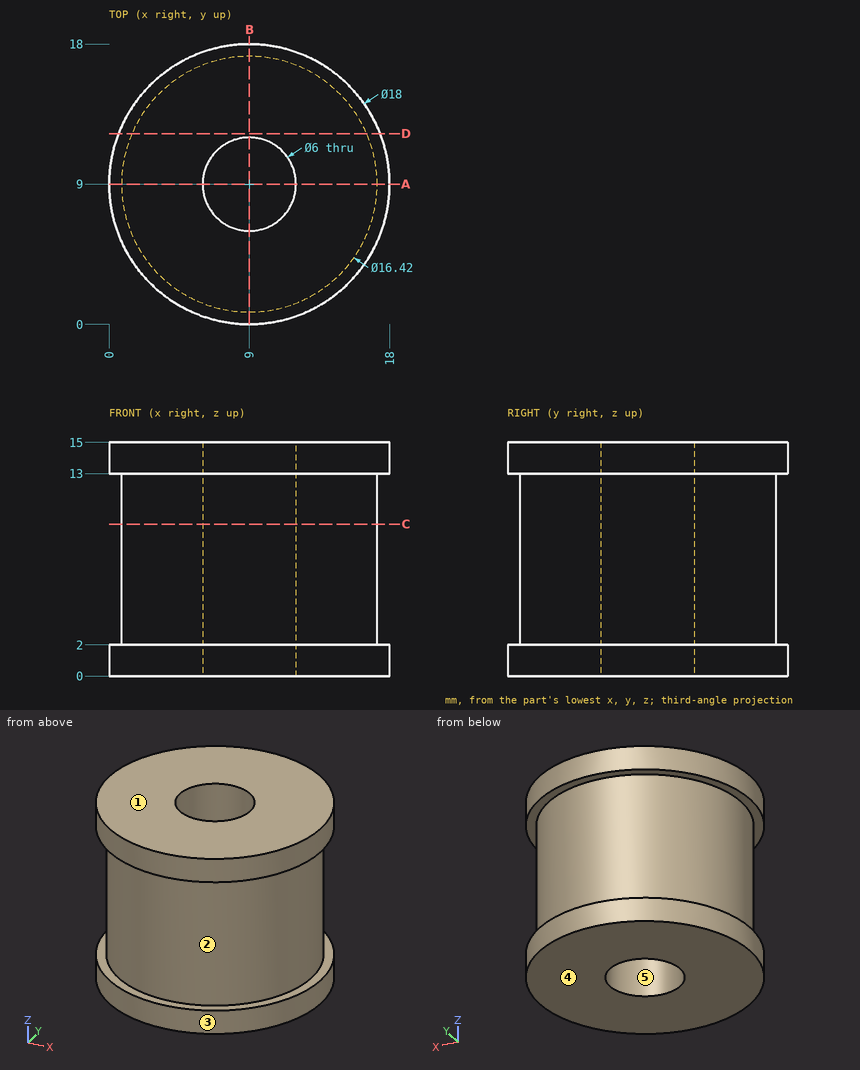
Answer from the drawing. Dimensions are ordinates in mm from the lowest x, y and z of the part. A direction names the side the tool comes from. Give positions to 0.01 mm unless a question says otherwise; leave off trailing zeros. Order: outer loops, then holes, each group sorted by start corner. A loop starts at its lowest first (then second) coordinate and runs counter-clockwise, first axis right, second up. Notation, with made-up numbers: (60.25, 55) -> (107.25, 55) arc R16 cw to (107.25, 74) -> close; hole circle Ø5 at (-29.75, 36). An arc over 180 degrees is marked (long way). One line per item, written item: value.
Item 1: Determine the mould class of the marked faces 3, 4 and 5 for opening direction X: released by +X, released by -X, zero draft, split by the parting line, or undercut.
Answer sheet:
face 3: split by the parting line
face 4: zero draft
face 5: undercut
Item 2: Straight lines are drawn through the part: probe 1 along Y at (x, z) = (9, 8.5); probe 2 along Z at (x, y) = (17.25, 5.5); probe 3 along Y at (x, z) = (10.75, 1.75). For each, find the intervals that lie inside material, in ascending order.
Answer sheet:
probe 1: 0.79 to 6, 12 to 17.21
probe 2: 0 to 2, 13 to 15
probe 3: 0.17 to 6.56, 11.44 to 17.83
Item 3: Find section C-C, the plane z = 9.75. Give the vertices of the cut face in (x, y), plus the area to 3 significant figures.
Answer sheet:
outline: circle Ø16.42 at (9, 9); hole circle Ø6 at (9, 9)
area: 183 mm²
Item 4: A tool of negligible diameter and unlimited length cuts with its end or side. For the marked faces 1 and 2, from which of +Z, -Z, +X, -X, +Y, -Y can it reach the whole face along a straight path? Write none if from no direction.
Answer sheet:
face 1: +Z, +X, -X, +Y, -Y
face 2: none
Item 5: Flat-ended cylindrical pins translate along their axes: P1, Ø1.5, axis at y = 10, z = 11, coming from the +X side; P2, Ø1.5, axis at x = 8, z = 3.5, coming from the -Y side; P3, Ø3, axis at y = 12, z = 4, coming from the +X side. Find the tip coordinate at first contact, or state that the pin passes through.
Answer sheet:
P1: x = 17.21
P2: y = 0.79
P3: x = 17.07
Item 6: Find section A-A, the plane y = 9. Give the vertices of the cut face in (x, z), plus the area to 3 significant figures.
Answer sheet:
outline: (0, 0) -> (6, 0) -> (6, 15) -> (0, 15) -> (0, 13) -> (0.79, 13) -> (0.79, 2) -> (0, 2) -> close; (12, 0) -> (18, 0) -> (18, 2) -> (17.21, 2) -> (17.21, 13) -> (18, 13) -> (18, 15) -> (12, 15) -> close
area: 163 mm²
Item 7: Find section D-D, the plane y = 12.25. Give the vertices of the cut face in (x, z), plus the area to 3 significant figures.
Answer sheet:
outline: (0.61, 0) -> (17.39, 0) -> (17.39, 2) -> (16.54, 2) -> (16.54, 13) -> (17.39, 13) -> (17.39, 15) -> (0.61, 15) -> (0.61, 13) -> (1.46, 13) -> (1.46, 2) -> (0.61, 2) -> close
area: 233 mm²
